Read the model definition and answer for the solid it produces. Units are mm, in the model's axes. Coordinates: 2 decimals unless noted, no trailing zeros. Write each loop counter-clockwise with the first axis right and the second up, starting at its lowest first coordinate (ties: lowest second). Pieces come first, ordered by that corner, then holes.
(1) Straight lines are drawn through the part: line 1 along X through (y, z) = (5.25, -12.7) (3 decimals); line 2 along X through (y, z) = (2.5, -13); line 3 along X through (y, z) = (5, -4). For each, find the intervals that lie inside material, in ascending order.
(2) The part is cut by section C-C, the plane y = 4.25. Determine the outline of the cut face in (x, z) (3 decimals), and give its area (3 significant figures).
(3) The part is cut by section A-A, the plane x = 25.4. Determine the outline of the cut face in (y, z).
(4) Given pin 1 (6 mm diameter, centred on x = 14, z = -10.5, fed in from -Y), flat-ended and moving along its own axis, determine where the tip first touches the part or whether it passes through.
(5) The part is cut by section B-B, the plane z = -12.7. Determine the outline of the cut face in (x, y) (3 decimals), and give its area (3 significant figures).
(6) Determine the mould class of faces 1 (the flat face through (0, 3, -13)), 2 (the cylindrical face through (58.55, 3.13, -4.5)), 3 (the flat face through (38, 3, -25.4)) for opening direction X: pulls with the +X half, pulls with the -X half, needs draft (parallel to the pull), parting line crosses it, or undercut.
(7) The part is cut by section D-D, the plane x = 57.15. Determine the outline of the cut face in (y, z) (3 decimals).
```python
from build123d import *

# Parameters (mm, degrees)
SKETCH2_W           = 76.2
SKETCH2_H           = 25.4
SKETCH2_R           = 1.41224
SKETCH2_R_2         = 1.905
BOSS_EXTRUDE1_DEPTH = 6.35
SKETCH3_R           = 2.0828
CUT_EXTRUDE1_DEPTH  = 6.35


with BuildPart() as part:
    # Sketch2 → Boss-Extrude1 (new body)
    with BuildSketch(Plane(origin=(0, 0, 0), x_dir=(1, 0, 0), z_dir=(0, 1, 0))):
        with Locations((38.1, 12.7)):
            Rectangle(SKETCH2_W, SKETCH2_H)
        with Locations(Location((57.15, 21.082, 0), (0, 0, 270))):
            Circle(SKETCH2_R, mode=Mode.SUBTRACT)
        with Locations(Location((57.15, 4.318, 0), (0, 0, 270))):
            Circle(SKETCH2_R, mode=Mode.SUBTRACT)
        with Locations(Location((57.15, 12.7, 0), (0, 0, 270))):
            Circle(SKETCH2_R_2, mode=Mode.SUBTRACT)
    extrude(amount=BOSS_EXTRUDE1_DEPTH)

    # Sketch3 → Cut-Extrude1 (cut)
    with BuildSketch(Plane(origin=(0, 6.35, 0), x_dir=(1, 0, 0), z_dir=(0, 1, 0))):
        with Locations(Location((25.4, 12.7, 0), (0, 0, 270))):
            Circle(SKETCH3_R)
    extrude(amount=-CUT_EXTRUDE1_DEPTH, mode=Mode.SUBTRACT)


solid = part.part
```
Computed:
1. line 1: x = 0 to 23.317, 27.483 to 55.245, 59.055 to 76.2
1. line 2: x = 0 to 23.34, 27.46 to 55.27, 59.03 to 76.2
1. line 3: x = 0 to 55.77, 58.53 to 76.2
2. outline: (0, -25.4) - (76.2, -25.4) - (76.2, 0) - (0, 0) - close; hole circle Ø4.166 at (25.4, -12.7); hole circle Ø3.81 at (57.15, -12.7); hole circle Ø2.824 at (57.15, -21.082); hole circle Ø2.824 at (57.15, -4.318)
2. area: 1,900 mm2
3. outline: (0, -25.4) - (6.35, -25.4) - (6.35, -14.78) - (0, -14.78) - close; (0, -10.62) - (6.35, -10.62) - (6.35, 0) - (0, 0) - close
4. pin 1: stops at y = 0
5. outline: (0, 0) - (23.317, 0) - (23.317, 6.35) - (0, 6.35) - close; (27.483, 0) - (55.245, 0) - (55.245, 6.35) - (27.483, 6.35) - close; (59.055, 0) - (76.2, 0) - (76.2, 6.35) - (59.055, 6.35) - close
5. area: 433 mm2
6. face 1: pulls with the -X half
6. face 2: undercut
6. face 3: needs draft
7. outline: (0, -25.4) - (6.35, -25.4) - (6.35, -22.494) - (0, -22.494) - close; (0, -19.67) - (6.35, -19.67) - (6.35, -14.605) - (0, -14.605) - close; (0, -10.795) - (6.35, -10.795) - (6.35, -5.73) - (0, -5.73) - close; (0, -2.906) - (6.35, -2.906) - (6.35, 0) - (0, 0) - close
